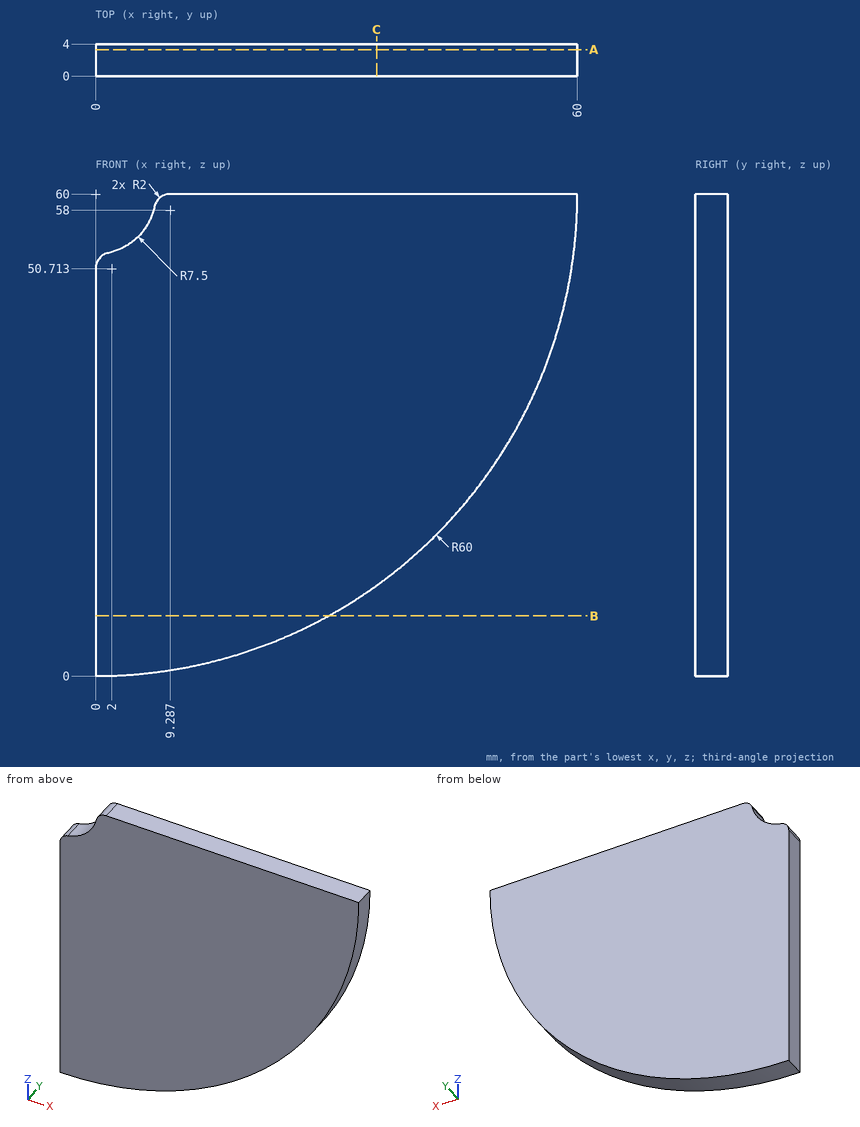
The drawing under review shows one solid part. Ordinate dimensions are in mm from its lowest x, y, z. Give positions to 0.01 mm unless a question says otherwise; leave off trailing zeros. Write each loop counter-clockwise with the first axis right and the second up, starting at its lowest first coordinate (ties: lowest second). Pieces come first, ordered by that corner, then holes. Notation, with made-up numbers: (81.5, -29) - (132.5, -29) arc R19 cw to (132.5, 4) - close; hole circle Ø3 at (74.5, -17.5). An arc over 180 degrees is marked (long way). Answer in a Markdown table with one row per item. Add a question column.
1. We need section C-C on x = 35. Write out the cut boundary in (y, z), then the cut area to 3 significant figures.
2. Wall thickness on line 1 along Z through (x, y) = (28, 3.05); line 2 along X through (y, z) = (1.6, 35); line 3 along Z through (x, y) = (13.5, 1.3): over which ranges is each line inside the solid? List them lowest first. Write a range as [from, to].
3. We need section B-B on z = 7.5. Write out the cut boundary in (x, y), then the cut area to 3 significant figures.
4. Insertion check: P1, Ø1, axis at y = 3.5, z = 54, coming from the +X side. The pin has a flat end and moves straight along its axis. Give the tip position at first contact, or say it passes through.
5. We need section A-A on y = 3.3. Write out the cut boundary in (x, z), then the cut area to 3 significant figures.
Ans:
| question | item | result |
|---|---|---|
| 1 | outline | (0, 11.27) - (4, 11.27) - (4, 60) - (0, 60) - close |
| 1 | area | 195 mm^2 |
| 2 | line 1 | z = [6.93, 60] |
| 2 | line 2 | x = [0, 54.54] |
| 2 | line 3 | z = [1.54, 60] |
| 3 | outline | (0, 0) - (29.05, 0) - (29.05, 4) - (0, 4) - close |
| 3 | area | 116 mm^2 |
| 4 | P1 | stops at x = 59.75 |
| 5 | outline | (0, 0) arc R60 ccw to (60, 60) - (9.29, 60) arc R2 ccw to (7.33, 58.42) arc R7.5 cw to (1.58, 52.67) arc R2 ccw to (0, 50.71) - close |
| 5 | area | 2,780 mm^2 |
